Autodesk Inventor part; units mm, degrees
ref_plane "YZ Plane" through (0, 0, 0) normal (1, 0, 0) x (0, 1, 0)
ref_plane "XZ Plane" through (0, 0, 0) normal (0, 1, 0) x (-1, 0, 0)
ref_plane "XY Plane" through (0, 0, 0) normal (0, 0, 1) x (1, 0, 0)
sketch "スケッチ1" plane through (0, 0, 0) normal (0, 1, 0) x (-1, 0, 0)
  line L0 (-40, -39) -> (40, -39)
  line L1 (40, -39) -> (40, 39)
  line L2 (40, 39) -> (-40, 39)
  line L3 (-40, 39) -> (-40, -39)
  line L4 (-40, -39) -> (40, 39) construction
  line L5 (40, -39) -> (-40, 39) construction
  point P0 (0, 0)
  dimension "d0" = 80
  dimension "d1" = 78
extrude "押し出し1" add sketch "スケッチ1" along normal blind 3
sketch "スケッチ2" plane through (0, 3, 0) normal (0, 1, 0) x (1, 0, 0)
  line L0 (34, 30) -> (-34, 30)
  line L1 (-34, 30) -> (-34, -30)
  line L2 (-34, -30) -> (34, -30)
  line L3 (34, -30) -> (34, 30)
  line L4 (34, 30) -> (-34, -30) construction
  line L5 (-34, 30) -> (34, -30) construction
  point P0 (0, 0)
  dimension "d4" = 68
  dimension "d5" = 60
hole "穴1" at (-34, 3, 30) at (34, 3, 30) at (34, 3, -30) at (-34, 3, -30) direction (0, -1, 0) diameter 5.2 depth 8 tip angle 118
sketch "スケッチ3" plane through (0, 3, 0) normal (0, 1, 0) x (1, 0, 0)
  line L0 (13.5, 25) -> (-13.5, 25)
  line L1 (-13.5, 25) -> (-13.5, -25)
  line L2 (-13.5, -25) -> (13.5, -25)
  line L3 (13.5, -25) -> (13.5, 25)
  line L4 (13.5, 25) -> (-13.5, -25) construction
  line L5 (-13.5, 25) -> (13.5, -25) construction
  point P0 (0, 0)
  dimension "d13" = 27
  dimension "d14" = 50
hole "穴2" at (-13.5, 3, 25) at (13.5, 3, 25) at (13.5, 3, -25) at (-13.5, 3, -25) direction (0, -1, 0) diameter 5.3 depth 8 tip angle 118 countersink diameter 11 countersink angle 90
sketch "スケッチ4" plane through (0, 0, 0) normal (0, -1, 0) x (1, 0, 0)
  line L0 (40, -39) -> (-40, -39)
  line L1 (26.3, -39) -> (63.5, -39)
  line L2 (63.5, -39) -> (63.5, 71)
  line L3 (63.5, 71) -> (26.3, 71)
  line L4 (26.3, 71) -> (26.3, -39)
  circle A0 centre (13.5, -25) radius 2.65
  circle A1 centre (-13.5, 25) radius 2.65
  circle A2 centre (13.5, 25) radius 2.65
  circle A3 centre (-13.5, -25) radius 2.65
  circle A4 centre (34, -30) radius 2.6
  circle A5 centre (-34, 30) radius 2.6
  circle A6 centre (34, 30) radius 2.6
  circle A7 centre (-34, -30) radius 2.6
  line L5 (-40, -39) -> (-40, 39)
  line L6 (40, -39) -> (-40, -39)
  line L7 (40, 39) -> (40, -39)
  line L8 (-40, 39) -> (40, 39)
  point P0 (0, 0)
  point P1 (26.3, 39)
  dimension "d23" = 110
  dimension "d24" = 50
extrude "押し出し2" add sketch "スケッチ4" against normal up to surface (3 mm away) contours L7 L8 L4 L3 L2 L1
sketch "スケッチ5" plane through (0, 3, 0) normal (0, 1, 0) x (1, 0, 0)
  circle A0 centre (13.5, 25) radius 5.5
  circle A1 centre (-13.5, -25) radius 5.5
  circle A2 centre (13.5, -25) radius 5.5
  circle A3 centre (-13.5, 25) radius 5.5
  circle A4 centre (34, 30) radius 2.6
  circle A5 centre (-34, -30) radius 2.6
  circle A6 centre (34, -30) radius 2.6
  circle A7 centre (-34, 30) radius 2.6
  line L0 (63.5, 39) -> (63.5, -71)
  line L1 (-40, 39) -> (63.5, 39)
  line L2 (-40, 39) -> (-40, -39)
  line L3 (-40, -39) -> (26.3, -39)
  line L4 (26.3, -71) -> (26.3, -39)
  line L5 (63.5, -71) -> (26.3, -71)
  point P0 (0, 0)
  point P1 (53.5, -59.5)
  point P2 (43.5, -59.5)
  dimension "d28" = 10
  dimension "d29" = 11.5
  dimension "d30" = 10
hole "穴3" at (53.5, 3, 59.5) at (43.5, 3, 59.5) direction (0, -1, 0) diameter 3.242 depth 11.8 tip angle 118
chamfer "面取り1" distance 20 angle 45 2 edges at (63.5, 1.5, -39) (26.3, 1.5, 39)
chamfer "面取り2" distance 5 angle 45 4 edges at (63.5, 1.5, 71) (26.3, 1.5, 71) (-40, 1.5, 39) (-40, 1.5, -39)
fillet "フィレット3" radius 2 12 edges at (63.5, 1.5, 66) (58.5, 1.5, 71) (31.3, 1.5, 71) (26.3, 1.5, 66) (26.3, 1.5, 59) (6.3, 1.5, 39) (-35, 1.5, 39) (-40, 1.5, 34) (-40, 1.5, -34) (-35, 1.5, -39) (63.5, 1.5, -19) (43.5, 1.5, -39)
properties part number "CCM_Mount_B"
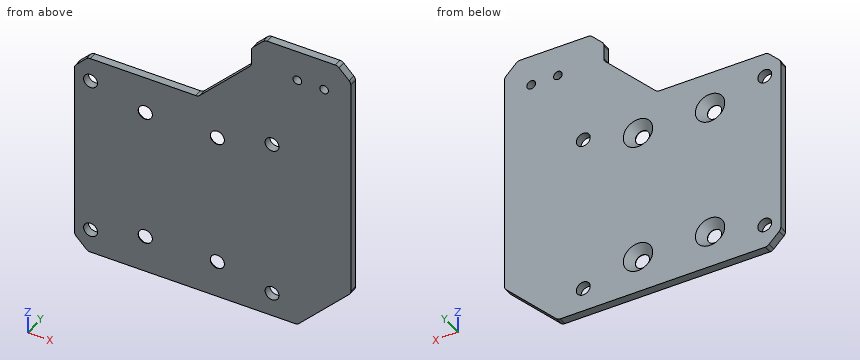
The listing builds one solid part. Answer for the finished solid, in the listing's coordinates (mm). Coordinates: 2 decimals unless noted, no trailing zeros. Write each loop counter-clockwise with the first axis right and the second up, starting at its lowest first coordinate (ties: lowest second). Pieces come first, ordered by that corner, then holes. Notation, with made-up numbers: M 12.5,22 L 34.5,22 A5 cw 34.5,29 Z; hole C 54.5,-21.5 d5. An arc over 180 degrees is marked long. Write each question's results on one line, items separated by ' | '.
Item 1: Consider probe 1 along X at (y, z) = (1.3, 30); probe 2 along X at (y, z) = (1.2, 59.5); probe 3 along Z at (x, y) = (-13.5, 0.1). Determine where each line is inside the solid, lowest interval first. Write a range as [from, to].
Answer below:
probe 1: [-40, -36.6], [-31.4, 31.4], [36.6, 63.5] | probe 2: [26.27, 41.88], [45.12, 51.88], [55.12, 63.5] | probe 3: [-39, -27.65], [-22.35, 22.35], [27.65, 39]
Item 2: Given P1, Ø8.5, axis at x = -13.5, z = 25, coming from the +Y side; P2, Ø3, axis at x = -34, z = -30, coming from the -Y side; P3, Ø0.9, axis at y = 1.5, z = 63, coming from the -X side; P4, Ø6, axis at x = 13.5, z = 25, coming from the +Y side, each flat-ended and moving along its own axis, determine where each tip first touches the part or whether it passes through.
Answer below:
P1: y = 1.75 | P2: through | P3: x = 26.3 | P4: y = 0.5
Item 3: The part is cut by section A-A on x = 13.5. Determine the outline of the cut face in (y, z), and give its area (3 significant figures).
Answer below:
outline: M 0,-39 L 3,-39 L 3,-30.5 L 0.15,-27.65 L 0,-27.65 Z; M 0,-22.35 L 0.15,-22.35 L 3,-19.5 L 3,19.5 L 0.15,22.35 L 0,22.35 Z; M 0,27.65 L 0.15,27.65 L 3,30.5 L 3,46.2 L 0,46.2 Z | area: 208 mm2
Item 4: The part is cut by section B-B on y = 1.5. State how many separate pieces and enclosed holes the cut face has, and give its area (3 significant figures).
Answer below:
separate pieces: 1 | enclosed holes: 10 | area: 8,910 mm2
Item 5: The part is cut by section D-D on z = -25. Determine the outline of the cut face in (x, y).
Answer below:
outline: M -40,0 L -16.15,0 L -16.15,0.15 L -19,3 L -40,3 Z; M -10.85,0 L 10.85,0 L 10.85,0.15 L 8,3 L -8,3 L -10.85,0.15 Z; M 16.15,0 L 57.5,0 L 57.5,3 L 19,3 L 16.15,0.15 Z
Item 6: The part is cut by section C-C on x = 53.5. Determine the outline of the cut face in (y, z), and give its area (3 significant figures).
Answer below:
outline: M 0,-29 L 3,-29 L 3,57.88 L 0,57.88 Z; M 0,61.12 L 3,61.12 L 3,71 L 0,71 Z | area: 290 mm2
